from build123d import *

# Parameters (mm, degrees)
SKETCH1_W                = 50
SKETCH1_H                = 40
BOSS_EXTRUDE1_DEPTH      = 25
BOSS_EXTRUDE2_DEPTH      = 20
BOSS_EXTRUDE2_DEPTH_BACK = 20
SKETCH2_R                = 37.5
CUT_EXTRUDE1_DEPTH       = 20
CUT_EXTRUDE1_DEPTH_BACK  = 20
SKETCH3_R                = 25


with BuildPart() as part:
    # Sketch1 → Boss-Extrude1 (new body)
    with BuildSketch(Plane(origin=(0, 0, 0), x_dir=(1, 0, 0), z_dir=(0, 1, 0))):
        Rectangle(SKETCH1_W, SKETCH1_H)
    extrude(amount=BOSS_EXTRUDE1_DEPTH)

    # Sketch2 → Boss-Extrude2 (add, two sides: drawn at the far end of the back side and taken through both)
    with BuildSketch(Plane.XY.offset(-BOSS_EXTRUDE2_DEPTH_BACK)):
        with Locations((0, 52.9)):
            Circle(SKETCH2_R)
    extrude(amount=BOSS_EXTRUDE2_DEPTH + BOSS_EXTRUDE2_DEPTH_BACK)

    # Sketch3 → Cut-Extrude1 (cut, two sides: drawn at the far end of the back side and taken through both)
    with BuildSketch(Plane.XY.offset(-CUT_EXTRUDE1_DEPTH_BACK)):
        with Locations((0, 52.9)):
            Circle(SKETCH3_R)
    extrude(amount=CUT_EXTRUDE1_DEPTH + CUT_EXTRUDE1_DEPTH_BACK, mode=Mode.SUBTRACT)


solid = part.part
Part model, mm, in its own coordinate system. A direction names the side the tool comes from. Round coordinates to 2 decimals unless told otherwise and drop trailing zeros. Write each loop counter-clockwise with the first axis right and the second up, starting at its lowest first coordinate (ties: lowest second). Pieces come first, ordered by that corner, then holes. Notation, with made-up numbers: (47, 73.25) - (87, 73.25) arc R10 cw to (87, 88.25) - close; hole circle Ø5 at (52.5, 8). An arc over 180 degrees is marked (long way). Use CSV: the item, a comma, the result in double quotes.
Item 1: Slice it at D-D, the plane x = 29. Write the cut outline in (y, z), then the cut area to 3 significant figures.
Results list:
outline,"(29.13, -20) - (76.67, -20) - (76.67, 20) - (29.13, 20) - close"
area,"1,900 mm²"
Item 2: Slice it at A-A, the plane x = 0. Write the cut outline in (y, z).
Results list:
outline,"(0, -20) - (27.9, -20) - (27.9, 20) - (0, 20) - close; (77.9, -20) - (90.4, -20) - (90.4, 20) - (77.9, 20) - close"
Item 3: Tool access for faces 4 (the flat face through (-25, 12, 0)), 5 (the flat face through (25, 12, 0)), 6 (the flat face through (0, 0, 0)): list every direction of +Z, -Z, +X, -X, +Y, -Y with a clear straight run to the whole face (end or side of a thin tool).
Results list:
face 4,"+Z, -Z, -X, -Y"
face 5,"+Z, -Z, +X, -Y"
face 6,"+Z, -Z, +X, -X, -Y"
Item 4: Wall check: L1, parallel to Y at x = 0.5, z = -6.5 (3 decimals); L2, parallel to X at y = 12.5, z = 0.5; L3, parallel to Y at x = 18, z = 7. Give the ranges that are in metal, low to high.
Results list:
L1,"y = 0 to 27.905, 77.895 to 90.397"
L2,"x = -25 to 25"
L3,"y = 0 to 35.55, 70.25 to 85.8"
Item 5: Slice it at C-C, the plane z = -7.5. Write the cut outline in (x, y), then the cut area to 3 significant figures.
Results list:
outline,"(-25, 0) - (25, 0) - (25, 24.95) arc R37.5 ccw (long way) to (-25, 24.95) - close; hole circle Ø50 at (0, 52.9)"
area,"3,370 mm²"
Item 6: Pull direction Y, two halves, no side cores. Call faces 1 (the flat face through (-1, 26, -20)), 2 (the cylindrical face through (-3.255, 77.687, -0.28)), 3 (the cylindrical face through (1.27, 90.38, -0.28)): pulls with the +Y half, pulls with the -Y half, needs draft (parallel to the pull), parting line crosses it, or undercut.
Results list:
face 1,"needs draft"
face 2,"undercut"
face 3,"parting line crosses it"
Item 7: Slice it at B-B, the plane y = 48.5. Write the cut outline in (x, z).
Results list:
outline,"(-37.24, -20) - (-24.61, -20) - (-24.61, 20) - (-37.24, 20) - close; (24.61, -20) - (37.24, -20) - (37.24, 20) - (24.61, 20) - close"
Item 8: Flat gauge pins, fed straight in: P1, Ø12.5, axis at y = 13.5, z = 4.5, coming from the -X side; P2, Ø12.5, axis at y = 9.5, z = -7, coming from the +X side; P3, Ø8, axis at x = 23, z = -1, coming from the -Y side; P4, Ø12, axis at y = 66.5, z = 3, coming from the +X side. Where does each tip first touch, or does it go through?
Results list:
P1,"stops at x = -25"
P2,"stops at x = 25"
P3,"stops at y = 0"
P4,"stops at x = 36.72"
